Could you check a few things on this model? Use its own coordinates, in mm. Round coordinates to 2 decimals unless told otherwise and drop trailing zeros. Return JSON: item names as keys, results as strings.
from build123d import *

# Parameters (mm, degrees)
SKETCH6_R          = 120
SKETCH6_R_2        = 100
CUT_EXTRUDE1_DEPTH = 74.5000001


with BuildPart() as part:
    # Sketch1 → Loft l3 section 0
    with BuildSketch(Plane(origin=(0, 0, 0), x_dir=(0, 0, -1), z_dir=(1, 0, 0))):
        Polygon((-73.5, 260), (53.5, 260), (53.5, 240), (0, 240), (0, -240), (53.5, -240), (53.5, -260), (-73.5, -260), (-73.5, -240), (-20, -240), (-20, 240), (-73.5, 240), align=None)
    # Sketch4 → Loft l3 section 1
    with BuildSketch(Plane(origin=(1250, 0, -1000), x_dir=(0, 0, 1), z_dir=(-1, 0, 0))):
        Polygon((967, 236), (1053, 236), (1053, 216), (1020, 216), (1020, -216), (1053, -216), (1053, -236), (967, -236), (967, -216), (1000, -216), (1000, 216), (967, 216), align=None)
    loft()

    # Sketch6 → Cut-Extrude1 (cut, through all)
    with BuildSketch(Plane.XY.offset(20)):
        with Locations((196.664397563, 0)):
            Circle(SKETCH6_R)
        with Locations((500.077852957, -3.284154434)):
            Circle(SKETCH6_R)
        with Locations((796.32876443, 0)):
            Circle(SKETCH6_R)
        with Locations((1070.806505034, 2.998831576)):
            Circle(SKETCH6_R_2)
    extrude(amount=-CUT_EXTRUDE1_DEPTH, mode=Mode.SUBTRACT)


solid = part.part
1) I want a section at A-A, the plane y = 49.5. Count the separate pieces of the cut face and the enclosed holes in it, and give its area (3 significant figures).
Return value:
{"separate pieces": "5", "enclosed holes": "0", "area": "8,400 mm²"}
2) Thinking about a two-plate mould opening in Y: for faces 1 (the face through (0, 1, 10)), 2 (the face through (76.78, 5.28, 10.14)), which applies, pulls with the +Y half, pulls with the -Y half, needs draft (parallel to the pull), parting line crosses it, or undercut?
Return value:
{"face 1": "needs draft", "face 2": "undercut"}
3) If I drill on probe 1 along X at (y, z) = (0, 12.25); probe 2 along X at (y, z) = (-56, 5.5); probe 3 along Z at (x, y) = (224.5, -171), over which ranges is the centre line in solid material (lowest first)? Write a range as [from, to].
Return value:
{"probe 1": "[0, 76.66], [316.66, 380.12], [620.03, 676.33], [916.33, 970.85], [1170.76, 1250]", "probe 2": "[0, 90.53], [302.8, 392.28], [607.88, 690.2], [902.46, 990.07], [1151.55, 1250]", "probe 3": "[0, 20]"}
4) Will these pins go through, and if not, where does the flat tip stop? pin 1 Ø12 at (x, y) = (767, 196.5) entering from -Z; pin 2 Ø3 at (x, y) = (324.5, -204) entering from +Z; pin 3 Ø1 at (x, z) = (847.5, 8.5) entering from -Y.
Return value:
{"pin 1": "z = 0", "pin 2": "z = 20", "pin 3": "y = -243.74"}
